Check sheet for the drawn part. Datum: minimum x, y, z corner. Units: mm. A direction names the side the tool comes from. Coordinates: 2 decimals unless noted, no trailing zeros. Loops run counter-clockwise (first coordinate to the right, second up) from the corner with the lowest first, then second, coordinate; pieces in that order, holes last. Notation, with made-up numbers: (67, 62) -> (106, 62) arc R23 cw to (106, 98) -> close; hole circle Ø9 at (-38.75, 34). An arc over 180 degrees is marked (long way). Use CSV: the item, a comma, the result in double quotes. Start each with the question number.
1. Gauge pin test, flat ends, axial feed: pin 1 (6.5 mm diameter, centred on x = 9, z = 21, fed in from +Y); pin 2 (8.5 mm diameter, centred on y = 14, z = 19, fed in from +X). Record the tip position at first contact, or that the pin passes through.
2. Sectioned sample at C-C, the plane y = 18. Record the cut outline in (x, z).
3. Thickness scan on L1, parallel to Y at x = 2.1, z = 15; L2, parallel to Y at x = 1.95, z = 7; L3, parallel to Y at x = 13, z = 11.75. Record the ranges inside material, lowest first.
4. Sectioned sample at A-A, the plane z = 15. Record the cut outline in (x, y).
5. Sectioned sample at D-D, the plane z = 22. Record the cut outline in (x, y).
6. Sectioned sample at B-B, the plane y = 11. Record the cut outline in (x, z).
7. Set-up check for the marked faces 1 and 2: record each of +Z, -Z, +X, -X, +Y, -Y from which the full face is reachable in a straight line by a thin tool's end or side.
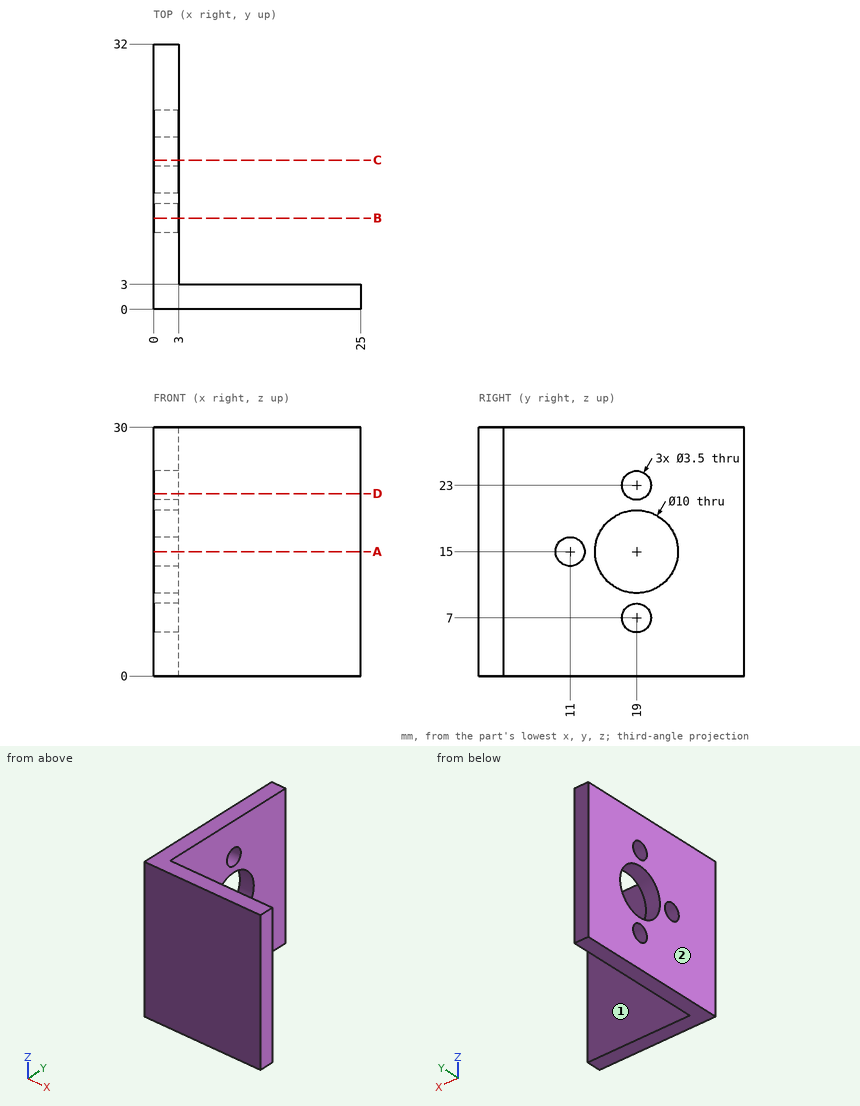
Completed:
1,pin 1,"y = 3"
1,pin 2,"x = 3"
2,outline,"(0, 0) -> (3, 0) -> (3, 5.56) -> (0, 5.56) -> close; (0, 8.44) -> (3, 8.44) -> (3, 10.1) -> (0, 10.1) -> close; (0, 19.9) -> (3, 19.9) -> (3, 21.56) -> (0, 21.56) -> close; (0, 24.44) -> (3, 24.44) -> (3, 30) -> (0, 30) -> close"
3,L1,"0 to 9.25, 12.75 to 14, 24 to 32"
3,L2,"0 to 17.25, 20.75 to 32"
3,L3,"0 to 3"
4,outline,"(0, 0) -> (25, 0) -> (25, 3) -> (3, 3) -> (3, 9.25) -> (0, 9.25) -> close; (0, 12.75) -> (3, 12.75) -> (3, 14) -> (0, 14) -> close; (0, 24) -> (3, 24) -> (3, 32) -> (0, 32) -> close"
5,outline,"(0, 0) -> (25, 0) -> (25, 3) -> (3, 3) -> (3, 17.56) -> (0, 17.56) -> close; (0, 20.44) -> (3, 20.44) -> (3, 32) -> (0, 32) -> close"
6,outline,"(0, 0) -> (3, 0) -> (3, 13.25) -> (0, 13.25) -> close; (0, 16.75) -> (3, 16.75) -> (3, 30) -> (0, 30) -> close"
7,face 1,"+Z, -Z, +X, +Y"
7,face 2,"+Z, -Z, -X, +Y, -Y"
